Autodesk Inventor part; units mm, degrees
ref_plane "Work Plane1" through (10, 0.5, -12.5) normal (0, -1, 0) x (1, 0, 0)
ref_plane "YZ Plane" through (0, 0, 0) normal (1, 0, 0) x (0, 1, 0)
ref_plane "XZ Plane" through (0, 0, 0) normal (0, 1, 0) x (-1, 0, 0)
sketch "Sketch1" plane through (0, 0, 0) normal (0, 1, 0) x (-1, 0, 0)
  line L0 (0, 0) -> (-30, 0)
  line L1 (-30, 0) -> (-30, -20)
  line L2 (-30, -20) -> (0, -20)
  line L3 (0, -20) -> (0, 0)
  dimension "d0" = 30
  dimension "d1" = 20
extrude "Plate1" add sketch "Sketch1" along normal blind 0.5
sketch "Sketch2" plane through (0, 0.5, 0) normal (0, 1, 0) x (1, 0, 0)
  arc A0 (5, 12.5) -> (10, 7.5) centre (10, 12.5) ccw
  line L0 (10, 7.5) -> (20, 7.5)
  arc A1 (20, 7.5) -> (25, 12.5) centre (20, 12.5) ccw
  line L1 (5, 12.5) -> (25, 12.5)
  line L2 (15, 12.5) -> (15, 7.5) construction
  line L3 (30, 0) -> (0, 0) construction
  line L4 (0, 0) -> (0, 20) construction
  point P0 (15, 10)
  dimension "d3" = 20
  dimension "d4" = 5
  dimension "d5" = 10
  dimension "d6" = 15
extrude "Extrusion1" cut sketch "Sketch2" against normal blind 0.5
ref_plane "Work Plane1" through (10, 0.5, -12.5) normal (0, -1, 0) x (1, 0, 0)
sketch "Sketch3" plane through (10, 0.5, -12.5) normal (0, -1, 0) x (1, 0, 0)
  arc A0 (0, 5) -> (-5, 0) centre (0, 0) ccw
  line L0 (-5, 0) -> (15, 0)
  line L1 (10, 5) -> (0, 5)
  arc A1 (15, 0) -> (10, 5) centre (10, 0) ccw
  line L2 (5, 0) -> (5, 5) construction
  line L3 (15, 0) -> (-5, 0)
  line L4 (-5, 0) -> (-5.5, 0)
  arc A2 (0, 5.5) -> (-5.5, 0) centre (0, 0) ccw
  line L5 (0, 5.5) -> (10, 5.5)
  arc A3 (15.5, 0) -> (10, 5.5) centre (10, 0) ccw
  line L6 (15.5, 0) -> (15, 0)
  point P0 (-10, 12.5)
  dimension "d9" = 0.5
revolve "Revolution1" add sketch "Sketch3" angle 90 about axis through (5, 0.5, -12.5) along (1, 0, 0) contours A0 L4 A2 L5 A3 L6 A1 L1
fillet "Fillet1" radius 1 6 edges at (6.4645, 0.5, -8.9645) (23.5355, 0.5, -8.9645) (15, 0.5, -7.5) (23.873, 0, -8.627) (6.127, 0, -8.627) (15, 0, -7.0228)
equation "\"d7\" = Thickness"
equation "\"d9\" = Thickness"
equation "\"d2\" = Thickness"
equation "\"BendRadius\" = Thickness"
equation "\"BendReliefWidth\" = Thickness"
equation "\"BendReliefDepth\" = 0.5 * Thickness"
equation "\"CornerReliefSize\" = 4 * Thickness"
equation "\"MinimumRemnant\" = 2 * Thickness"
equation "\"TransitionRadius\" = BendRadius"
equation "\"JacobiRadiusSize\" = BendRadius"
equation "\"GapSize\" = Thickness"
properties part number "CE-4.1.2"
Can you work these out from the model? Positions are in its coordinate system, mm. Round coordinates to 2 decimals unless told otherwise and drop trailing zeros. Loops run counter-clockwise (first coordinate to the right, second up) from the corner with the lowest first, then second, coordinate; pieces in that order, holes last. Notation, with made-up numbers: M 84,-32 L 127,-32 A17 cw 127,-18 Z; hole C 77.5,10 d11. An arc over 180 degrees is marked long. Write item = value, one per line. Start each with the question number.
(1) Suppose I cut it at B-B on y = -2.15. Write out the boundary of the cut face in (x, z).
(2) If we mould it in two halves opening along X, with no side actions, what happens to faces 1 (the face through (14.93, -3.35, -9.31)), 2 (the face through (14.93, 0.27, -7.22)), 3 (the face through (14.9, -4.7, -12.5))? For each: released by +X, released by -X, zero draft, split by the parting line, or undercut.
(3) Suppose I cut it at C-C on z = -16.75. Write out the boundary of the cut face in (x, y), plus the area to 3 significant figures.
(4) Suppose I cut it at D-D on y = -3.6. Write out the boundary of the cut face in (x, z), plus the area to 3 significant figures.
(5) I need wall thicknesses on line 1 along Y through (x, z) = (27.25, -10); line 2 along X through (y, z) = (-2, -8.75); line 3 along Z through (x, y) = (23, 0.25). Which ranges of each line are inside material? Lowest first, please.
(6) I'm going to push flat-ended pins straight in: P1, Ø2.5, axis at x = 17, y = -3.5, coming from the -Z side; P2, Ø3, axis at x = 6.5, y = -4, coming from the +Z side; P3, Ø0.6, axis at x = 11, y = 0.5, coming from the +Z side. Where does each tip first touch, or does it pass through?
(7) Suppose I cut it at A-A on x = 10.5. Write out the boundary of the cut face in (y, z).
Answer block:
q1.outline = M 5.18,-12.5 L 5.76,-12.5 A4.24 cw 10,-8.26 L 20,-8.26 A4.24 cw 24.24,-12.5 L 24.82,-12.5 A4.82 ccw 20,-7.68 L 10,-7.68 A4.82 ccw Z
q2.face_1 = undercut
q2.face_2 = undercut
q2.face_3 = zero draft
q3.outline = M 0,0 L 30,0 L 30,0.5 L 0,0.5 Z
q3.area = 15.0 mm²
q4.outline = M 6.33,-12.5 L 7.14,-12.5 A2.86 cw 10,-9.64 L 20,-9.64 A2.86 cw 22.86,-12.5 L 23.67,-12.5 A3.67 ccw 20,-8.83 L 10,-8.83 A3.67 ccw Z
q4.area = 16.3 mm²
q5.line_1 = 0 to 0.5
q5.line_2 = 6.85 to 7.83, 22.17 to 23.15
q5.line_3 = -20 to -12.5, -8.19 to 0
q6.P1 = -12.5
q6.P2 = -8.95
q6.P3 = 0
q7.outline = M -5,-12.5 L -4.5,-12.5 A5 cw -0.33,-7.57 A1 ccw 0.5,-6.58 L 0.5,0 L 0,0 L 0,-6.18 A1 cw -0.77,-7.15 A5.5 ccw Z; M 0,-20 L 0.5,-20 L 0.5,-12.5 L 0,-12.5 Z
